from build123d import *

# Parameters (mm, degrees)
F1_DEPTH = 98.806
F3_DEPTH = 80.772


with BuildPart() as f1:
    # F0 (on Front) → F1 (new body)
    with BuildSketch(Plane.XZ):
        Polygon((0, -20.002501), (24.888605, -60.007501), (12.062577, 0), (38.630784, -31.607002), (12.062577, 30.080097), (24.888605, 71.306624), (0, 30.080097), (-23.66708, 71.306624), (-11.757195, 30.080097), (-43.516889, -31.607002), (-11.757195, 0), (-18.780975, -58.480591), align=None)
    extrude(amount=-F1_DEPTH)

    # F2 (on face) → F3 (cut)
    with BuildSketch(Plane.XZ):
        Polygon((8.546956, 29.895244), (13.65233, 46.305379), (-0.071587, 23.572508), (-12.891517, 45.904), (-8.220637, 29.735567), (-30.981843, -14.473698), (-7.34452, 9.049982), (-13.170568, -39.45819), (-0.349297, -13.190223), (17.709537, -42.21731), (6.063784, 12.268189), (26.72525, -12.311829), align=None)
    extrude(amount=-F3_DEPTH, mode=Mode.SUBTRACT)


solid = f1.part
The listing builds one solid part. Answer for the finished solid, in the listing's coordinates (mm). A direction names the side the tool comes from. Give positions to 0.01 mm unless a question says otherwise; leave off trailing zeros. Loops run counter-clockwise (first coordinate to the right, second up) from the corner with the lowest first, then second, coordinate; pieces in that order, holes last. Notation, with made-up numbers: (68, -39.5) - (80, -39.5) arc R26 ccw to (80, -22.5) - close; hole circle Ø2 at (48.25, 75). An arc over 180 degrees is marked (long way). Answer as a JSON object with one key per item and string values.
1. Find the intervals of material crossed by L1, parallel to X at y = 13, z = 34; L2, parallel to X at y = 35, z = 5.5; L3, parallel to X at y = 24, z = -11, in increasing order. Write a range as [from, to].
Determined:
{"L1": "[-12.89, -9.45], [-6.06, -2.25], [2.37, 6.22], [9.82, 13.28]", "L2": "[-24.41, -20.7], [-10.91, -7.77], [7.51, 11.75], [19.05, 22.65]", "L3": "[-32.91, -29.19], [-27.49, -22.81], [-13.08, -9.75], [11.04, 14.41], [21.31, 25.62], [26.16, 29.76]"}
2. A cutting plane is placed at A-A (y = 21). Write down the section's boundary in (x, z).
Determined:
{"outline": "(-43.52, -31.61) - (-11.76, 0) - (-18.78, -58.48) - (0, -20) - (24.89, -60.01) - (12.06, 0) - (38.63, -31.61) - (12.06, 30.08) - (24.89, 71.31) - (0, 30.08) - (-23.67, 71.31) - (-11.76, 30.08) - close; hole (-30.98, -14.47) - (-7.34, 9.05) - (-13.17, -39.46) - (-0.35, -13.19) - (17.71, -42.22) - (6.06, 12.27) - (26.73, -12.31) - (8.55, 29.9) - (13.65, 46.31) - (-0.07, 23.57) - (-12.89, 45.9) - (-8.22, 29.74) - close"}
3. A cutting plane is placed at C-C (y = 84). Write down the section's boundary in (x, z), then the cut area to 3 significant figures.
Determined:
{"outline": "(-43.52, -31.61) - (-11.76, 0) - (-18.78, -58.48) - (0, -20) - (24.89, -60.01) - (12.06, 0) - (38.63, -31.61) - (12.06, 30.08) - (24.89, 71.31) - (0, 30.08) - (-23.67, 71.31) - (-11.76, 30.08) - close", "area": "3,230 mm²"}
4. Flat-ended cylindrical pins translate along their axes: pin 1 Ø4 at (y, z) = (45.5, 47) entering from -X; pin 2 Ø3 at (x, y) = (16, 19) entering from +Z; pin 3 Ø8 at (x, z) = (26, 16.5) entering from +Y; pin 4 Ø4 at (x, y) = (-14.5, 85.5) entering from +Z. Find the tip coordinate at first contact, or state that the pin passes through.
Determined:
{"pin 1": "x = -17.22", "pin 2": "z = 59.07", "pin 3": "through", "pin 4": "z = 58.82"}
5. For a pull along Z with two mould halves and no side action, classify faces 1 (the flat face through (-3, 98.806, 1)), 2 (the flat face through (-9.52, 48.71, -39.51)), 3 (the flat face through (-6.85, 39.82, -26.51)) as pulls with the +Z half, pulls with the -Z half, needs draft (parallel to the pull), parting line crosses it, or undercut.
Determined:
{"face 1": "needs draft", "face 2": "pulls with the -Z half", "face 3": "undercut"}
6. A cutting plane is placed at B-B (z = 49). Write down the section's boundary in (x, y), then the cut area to 3 significant figures.
Determined:
{"outline": "(-17.22, 0) - (-10.86, 0) - (-10.86, 98.81) - (-17.22, 98.81) - close; (11.42, 0) - (17.95, 0) - (17.95, 98.81) - (11.42, 98.81) - close", "area": "1,270 mm²"}
7. For faces 4 (the flat face through (-27.859, 48.711, -16.025)), 5 (the flat face through (25.533, 48.711, -1.195)), 6 (the flat face through (-17.8, 48.7, 51)), 7 (the flat face through (-10.217, 39.821, -14.865)), determine the directions among +Z, -Z, +X, -X, +Y, -Y from which every point of the face is accessible in a straight line to the end or side of a thin tool.
Determined:
{"face 4": "+Y, -Y", "face 5": "+X, +Y, -Y", "face 6": "-X, +Y, -Y", "face 7": "-Y"}
8. A cutting plane is placed at D-D (x = -22). Write down the section's boundary in (y, z).
Determined:
{"outline": "(0, -10.19) - (98.81, -10.19) - (98.81, 10.19) - (0, 10.19) - (0, 2.97) - (80.77, 2.97) - (80.77, -5.54) - (0, -5.54) - close; (0, 65.54) - (98.81, 65.54) - (98.81, 68.4) - (0, 68.4) - close"}
